Geometry: see drawing. Coordinates: mm, zero at the bounding-box minimum. Coordinates: 2 decimals unless noted, no trailing zeros. Write each loop counter-clockwise with the first axis right and the second up, starting at its lowest first coordinate (ties: lowest second). Pieces come first, ordered by that corner, then holes. Notation, with made-up numbers: (49, -16) - (71, -16) arc R18 cw to (71, 8) - close; hole circle Ø4 at (-39.75, 21). An arc over 180 degrees is marked (long way). Use CSV: the item, a comma, the result in double quotes.
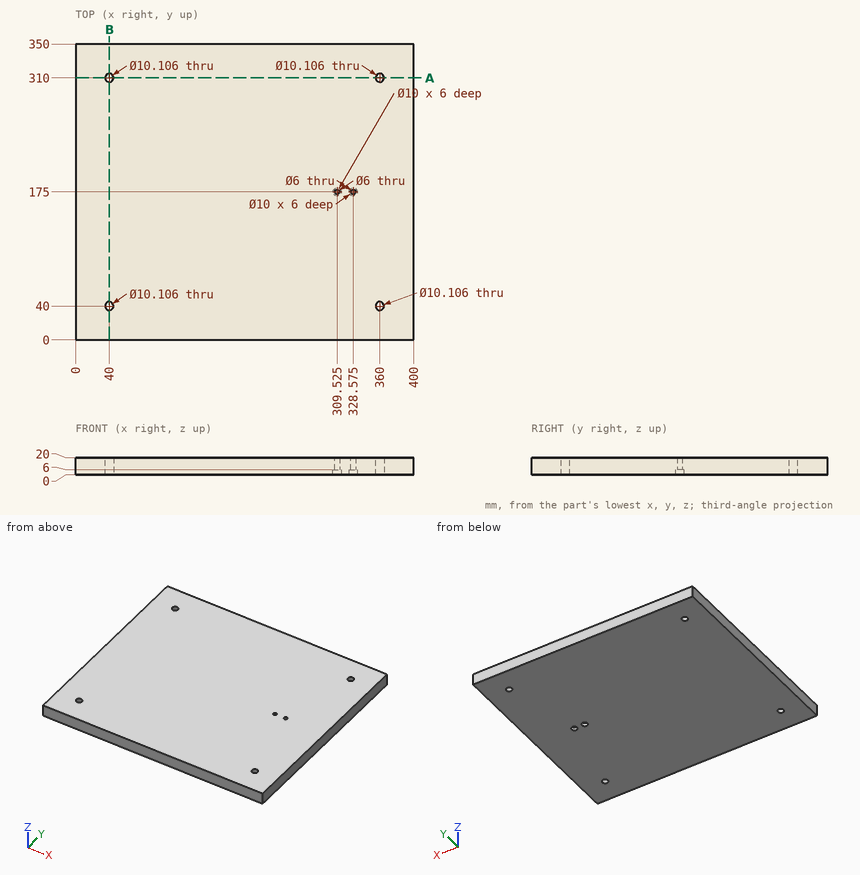
(1) Cut plane A-A on y = 310. Return loops of the section in (x, z), and give its area (3 significant figures).
Check values:
outline,"(0, 0) - (34.95, 0) - (34.95, 20) - (0, 20) - close; (45.05, 0) - (354.95, 0) - (354.95, 20) - (45.05, 20) - close; (365.05, 0) - (400, 0) - (400, 20) - (365.05, 20) - close"
area,"7,600 mm^2"
(2) Cut plane B-B on x = 40. Return loops of the section in (y, z), and give its area (3 significant figures).
Check values:
outline,"(0, 0) - (34.95, 0) - (34.95, 20) - (0, 20) - close; (45.05, 0) - (304.95, 0) - (304.95, 20) - (45.05, 20) - close; (315.05, 0) - (350, 0) - (350, 20) - (315.05, 20) - close"
area,"6,600 mm^2"
(3) Pin query (flat end, axial travel): pin 1 Ø7 at (x, y) = (328.575, 175) entering from -Z; pin 2 Ø9 at (x, y) = (40, 310) entering from +Z. Return the tip coordinate at first contact, or that it passes through.
Check values:
pin 1,"z = 6"
pin 2,"through"
(4) Ray query, probe 1 along X at (y, z) = (310, 7.25); probe 2 along X at (y, z) = (311, 16). Return the intervals inside material, ascending. Write a range as from..to.
Check values:
probe 1,"0..34.95, 45.05..354.95, 365.05..400"
probe 2,"0..35.05, 44.95..355.05, 364.95..400"
